The model under review builds one solid part; all positions refer to its coordinate system, in mm. A direction names the side the tool comes from. Coordinates: 2 decimals unless noted, no trailing zeros. Order: outer loops, then holes, each group sorted by start corner. A loop starts at its lowest first (then second) coordinate and runs counter-clockwise, first axis right, second up. Notation, with made-up numbers: (5, 46) -> (45, 46) arc R7 cw to (45, 54) -> close; hole circle Ø2 at (-28, 67.5). An arc over 180 degrees is marked (long way). Use one line per item in the form item = value.
from build123d import *

# Parameters (mm, degrees)
SKETCH_1_R      = 2.4
EXTRUDE_1_DEPTH = 40
SKETCH_2_R      = 2.5
EXTRUDE_2_DEPTH = 10


with BuildPart() as part:
    # 草图1 → 凸台-拉伸1 (new body)
    with BuildSketch(Plane(origin=(0, 0, 0), x_dir=(1, 0, 0), z_dir=(0, 1, 0))):
        with Locations(Location((0, 0, 0), (0, 0, 270))):
            Circle(SKETCH_1_R)
    extrude(amount=EXTRUDE_1_DEPTH)

    # 草图2 → 凸台-拉伸2 (add, symmetric)
    with BuildSketch(Plane(origin=(0, 20, 0), x_dir=(-1, 0, 0), z_dir=(0, -1, 0))):
        with Locations(Location((0, 0, 0), (0, 0, 90))):
            Circle(SKETCH_2_R)
    extrude(amount=EXTRUDE_2_DEPTH, both=True)


solid = part.part
Item 1: To check wall thickness, follow L1, parallel to Z at x = 0.1, y = 16; L2, parallel to Y at x = -2.1, z = 1.3. State the ranges of each line that lie inside material, in increasing order. Write a range as from..to.
Results found:
L1 = -2.5..2.5
L2 = 10..30
Item 2: We need section A-A (x = 0). Write out the cut boundary in (y, z), plus the area to 3 significant figures.
Results found:
outline = (0, -2.4) -> (10, -2.4) -> (10, -2.5) -> (30, -2.5) -> (30, -2.4) -> (40, -2.4) -> (40, 2.4) -> (30, 2.4) -> (30, 2.5) -> (10, 2.5) -> (10, 2.4) -> (0, 2.4) -> close
area = 196 mm²
Item 3: We need section C-C (y = 36.5). Write out the cut boundary in (x, z), plus the area to 3 significant figures.
Results found:
outline = circle Ø4.8 at (0, 0)
area = 18.1 mm²
Item 4: Tool access review of faces 1 (the face through (2.024, 34.93, 1.29)), 2 (the face through (0, 40, 0)), 3 (the face through (2.024, 4.93, 1.29)): name each direction out of +Z, -Z, +X, -X, +Y, -Y from which nothing blocks a thin tool from reaching the whole face with its end or side.
Results found:
face_1 = +Y
face_2 = +Z, -Z, +X, -X, +Y
face_3 = -Y
Item 5: Clearance check with a flat-ended pin moving along its axis: pin 1 (2 mm diameter, centred on y = 5.5, z = 1.5, fed in from -X). State where the tip first meets the part, or that it passes through.
Results found:
pin_1 = -2.35
Item 6: We need section B-B (z = 0). Write out the cut boundary in (x, y), plus the area to 3 significant figures.
Results found:
outline = (-2.5, 10) -> (-2.4, 10) -> (-2.4, 0) -> (2.4, 0) -> (2.4, 10) -> (2.5, 10) -> (2.5, 30) -> (2.4, 30) -> (2.4, 40) -> (-2.4, 40) -> (-2.4, 30) -> (-2.5, 30) -> close
area = 196 mm²
Item 7: We need section D-D (y = 19). Write out the cut boundary in (x, z), plus the area to 3 significant figures.
Results found:
outline = circle Ø5 at (0, 0)
area = 19.6 mm²
